Here's how the part is built. I have some questions about the finished solid (model axes, mm). Face numbers are marked on the shaded views. A direction names the side the tool comes from. Round coordinates to 2 decimals unless told otherwise and drop trailing zeros. Order: outer loops, then holes, each group sorted by start corner. A loop starts at its lowest first (then second) coordinate and runs counter-clockwise, first axis right, second up. Notation, with made-up numbers: M -3.75,23 L 49.25,23 A12 ccw 49.25,34 Z; hole C -6,24.5 d4. An arc over 180 degrees is marked long. Use one line per item in the form item = value. Start each with the question number.
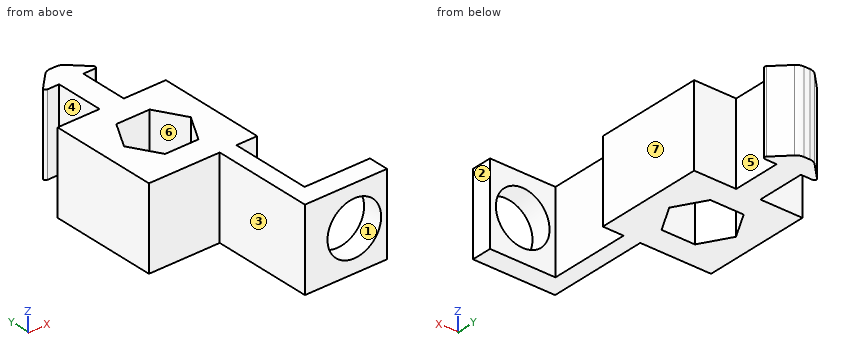
```python
from build123d import *

# Parameters (mm, degrees)
BOSS_EXTRUDE1_DEPTH = 10.16
SKETCH3_W           = 4.197769469
SKETCH3_H           = 20.32
BOSS_EXTRUDE2_DEPTH = 25.4
SKETCH4_W           = 16.450422122
SKETCH4_H           = 20.32
SKETCH4_R           = 6.75
BOSS_EXTRUDE3_DEPTH = 5.08


with BuildPart() as part:
    # Sketch1 → Boss-Extrude1 (new, symmetric)
    with BuildSketch(Plane.XY):
        with BuildLine():
            Line((-13.62075, 13.62075), (-13.62075, -13.62075))
            Line((-13.62075, -13.62075), (13.62075, -13.62075))
            Line((13.62075, -13.62075), (13.62075, 13.62075))
            Line((13.62075, 13.62075), (3.048, 13.62075))
            Line((3.048, 13.62075), (3.048, 25.68575))
            Line((3.048, 25.68575), (6.01257951, 25.68575))
            ThreePointArc((6.01257951, 25.68575), (6.481910313, 25.999346816), (6.371789755, 26.552960245))
            Line((6.371789755, 26.552960245), (2.532108776, 30.392641224))
            ThreePointArc((2.532108776, 30.392641224), (1.70807347, 30.943244013), (0.736057552, 31.13659))
            Line((0.736057552, 31.13659), (-0.736057552, 31.13659))
            ThreePointArc((-0.736057552, 31.13659), (-1.70807347, 30.943244013), (-2.532108776, 30.392641224))
            Line((-2.532108776, 30.392641224), (-6.371789755, 26.552960245))
            ThreePointArc((-6.371789755, 26.552960245), (-6.481910313, 25.999346816), (-6.01257951, 25.68575))
            Line((-6.01257951, 25.68575), (-3.048, 25.68575))
            Line((-3.048, 25.68575), (-3.048, 13.62075))
            Line((-3.048, 13.62075), (-13.62075, 13.62075))
        make_face()
        Polygon((-4.19776947, 7.27075), (-8.395538939, 0), (-4.19776947, -7.27075), (4.19776947, -7.27075), (8.395538939, 0), (4.19776947, 7.27075), align=None, mode=Mode.SUBTRACT)
    extrude(amount=BOSS_EXTRUDE1_DEPTH, both=True)

    # Sketch3 → Boss-Extrude2 (add)
    with BuildSketch(Plane.XZ.offset(13.62075)):
        with Locations((6.296654204, 0)):
            Rectangle(SKETCH3_W, SKETCH3_H)
    extrude(amount=BOSS_EXTRUDE2_DEPTH)

    # Sketch4 → Boss-Extrude3 (add)
    with BuildSketch(Plane.XZ.offset(39.02075)):
        with Locations((16.62075, 0)):
            Rectangle(SKETCH4_W, SKETCH4_H)
        with Locations(Location((16.62075, 0, 0), (0, 0, 270))):
            Circle(SKETCH4_R, mode=Mode.SUBTRACT)
    extrude(amount=-BOSS_EXTRUDE3_DEPTH)


solid = part.part
```
1) If we section it at C-C on x = 0: Write out the boundary of the cut face in (y, z).
2) Will these pins go through, and if not, where does the flat tip stop? pin 1 Ø1 at (x, z) = (-8, -6) entering from -Y; pin 2 Ø9.5 at (y, z) = (21.5, 5) entering from +X; pin 3 Ø12 at (x, y) = (20.5, -9) entering from +Z; pin 4 Ø8 at (y, z) = (2.5, -7) entering from +X.
3) On a 3-axis mill with a long thin cutter (end or side, diameter ignored), from which of +Z, -Z, +X, -X, +Y, -Y can I reach the whole of each face in a straight line? I mean the marked faces 4, 5, 6 and 7. Say none if no direction works.
4) If we section it at A-A on z = 0: Give the number of separate pieces and of enclosed holes in the cut face, then the cut area to 3 significant figures.
5) If we mould it in two halves opening along X, with no side actions, what happens to the marked faces 1, 2 and 3? For each: +X half, -X half, draft (parallel to the pull), parting line (faces both ways), or undercut.
6) If we section it at B-B on x = -5: Write out the boundary of the cut face in (y, z).
7) If I drill on line 1 (X direction, y = -37.3, z = 0); line 2 (Y direction, x = 3.5, z = -8.5); line 3 (Y direction, x = 10.5, z = -5), over which ranges is the centre line in solid material (lowest first)?
Completed:
q1.outline = M -13.62,-10.16 L -7.27,-10.16 L -7.27,10.16 L -13.62,10.16 Z; M 7.27,-10.16 L 31.14,-10.16 L 31.14,10.16 L 7.27,10.16 Z
q2.pin_1 = -13.62
q2.pin_2 = 6.52
q2.pin_3 = through
q2.pin_4 = 13.62
q3.face_4 = +Z, -Z, -X
q3.face_5 = +Z, -Z, +X
q3.face_6 = +Z, -Z
q3.face_7 = +Z, -Z, +X, +Y
q4.separate_pieces = 2
q4.enclosed_holes = 1
q4.area = 802 mm²
q5.face_1 = undercut
q5.face_2 = +X half
q5.face_3 = -X half
q6.outline = M -13.62,-10.16 L -5.88,-10.16 L -5.88,10.16 L -13.62,10.16 Z; M 5.88,-10.16 L 13.62,-10.16 L 13.62,10.16 L 5.88,10.16 Z; M 25.69,-10.16 L 27.92,-10.16 L 27.92,10.16 L 25.69,10.16 Z
q7.line_1 = 4.2 to 9.87, 23.37 to 24.85
q7.line_2 = -13.62 to -7.27, 7.27 to 13.62, 25.69 to 29.42
q7.line_3 = -39.02 to -33.94, -13.62 to 13.62
